Autodesk Inventor part; units mm, degrees
ref_plane "YZ Plane" through (0, 0, 0) normal (1, 0, 0) x (0, 1, 0)
ref_plane "XZ Plane" through (0, 0, 0) normal (0, 1, 0) x (-1, 0, 0)
ref_plane "XY Plane" through (0, 0, 0) normal (0, 0, 1) x (1, 0, 0)
sketch "Sketch1" plane through (0, 0, 0) normal (0, 0, 1) x (1, 0, 0)
  line L0 (0, 0) -> (0, 33)
  line L1 (0, 33) -> (19, 33)
  line L2 (19, 33) -> (19, 0)
  line L3 (19, 0) -> (0, 0)
  dimension "d0" = 33
  dimension "d1" = 19
extrude "Extrusion1" add sketch "Sketch1" along normal blind 4
sketch "Sketch2" plane through (0, 33, 0) normal (0, 1, 0) x (1, 0, 0)
  line L0 (19, 0) -> (0, 0)
  line L1 (19, 0) -> (19, -24)
  line L2 (19, -24) -> (15, -24)
  line L3 (15, -24) -> (15, 0)
  line L4 (15, 0) -> (19, 0)
  dimension "d4" = 24
  dimension "d5" = 4
  dimension "d6" = 24
extrude "Extrusion2" add sketch "Sketch2" against normal blind 33
sketch "Sketch3" plane through (0, 33, 0) normal (0, 1, 0) x (1, 0, 0)
  line L0 (15, -4) -> (15, -24)
  line L1 (15, -24) -> (95, -24)
  line L2 (95, -24) -> (95, -20)
  line L3 (95, -20) -> (15, -20)
  line L4 (15, -20) -> (15, -24)
  point P0 (0, 0)
  dimension "d9" = 80
  dimension "d10" = 4
  dimension "d11" = 80
extrude "Extrusion3" add sketch "Sketch3" against normal blind 33
sketch "Sketch4" plane through (0, 33, 0) normal (0, 1, 0) x (1, 0, 0)
  line L0 (15, -24) -> (95, -24)
  line L1 (95, -24) -> (95, 0)
  line L2 (95, 0) -> (91, 0)
  line L3 (91, 0) -> (91, -24)
  line L4 (91, -24) -> (95, -24)
  point P0 (0, 0)
  dimension "d14" = 24
  dimension "d15" = 4
  dimension "d16" = 24
extrude "Extrusion4" add sketch "Sketch4" against normal blind 33
sketch "Sketch5" plane through (0, 33, 0) normal (0, 1, 0) x (1, 0, 0)
  line L0 (91, 0) -> (91, -20)
  line L1 (91, 0) -> (110, 0)
  line L2 (110, 0) -> (110, -4)
  line L3 (110, -4) -> (91, -4)
  line L4 (91, -4) -> (91, 0)
  point P0 (0, 0)
  dimension "d19" = 19
  dimension "d20" = 4
  dimension "d21" = 19
  dimension "d22" = 4
extrude "Extrusion5" add sketch "Sketch5" against normal blind 33
sketch "Sketch6" plane through (15, 0, 24) normal (0, 0, 1) x (1, 0, 0)
  line L0 (80, 33) -> (80, 0)
  line L1 (30, 33) -> (30, 22.18)
  line L2 (50, 33) -> (50, 22.18)
  arc A0 (30.0006, 22.18) -> (49.9994, 22.18) centre (40, 16.5) ccw
  line L3 (30, 22.18) -> (30.0006, 22.18)
  line L4 (49.9994, 22.18) -> (50, 22.18)
  line L5 (30, 33) -> (50, 33)
  line L6 (0, 33) -> (80, 33)
  point P0 (-15, 0)
  dimension "d27" = 10.82
  dimension "d28" = 10.82
  dimension "d30" = 23
extrude "Extrusion6" cut sketch "Sketch6" against normal blind 4
sketch "Sketch7" plane through (0, 0, 0) normal (0, 0, -1) x (-1, 0, 0)
  line L0 (0, 33) -> (-19, 33)
  line L1 (-19, 0) -> (0, 0)
  circle A0 centre (-9.5, 24.5) radius 2.5
  circle A1 centre (-9.5, 8.5) radius 2.5
  dimension "d35" = 5
  dimension "d36" = 5
extrude "Extrusion7" cut sketch "Sketch7" against normal blind 4
sketch "Sketch8" plane through (91, 0, 0) normal (0, 0, -1) x (-1, 0, 0)
  circle A0 centre (-9.5, 24.5) radius 2.5
  circle A1 centre (-9.5, 8.5) radius 2.5
  point P0 (91, 0)
  point P1 (-19, 33)
  point P2 (0, 33)
  point P3 (-19, 0)
  point P4 (0, 0)
  dimension "d39" = 19
  dimension "d43" = 5
  dimension "d44" = 5
extrude "Extrusion8" cut sketch "Sketch8" against normal blind 4
sketch "Sketch9" plane through (15, 0, 24) normal (0, 0, 1) x (1, 0, 0)
  line L0 (0, 33) -> (30, 33)
  line L1 (0, 0) -> (0, 33)
  circle A0 centre (22.5, 16.5) radius 2.5
  line L2 (50, 33) -> (80, 33)
  line L3 (80, 0) -> (80, 33)
  circle A1 centre (57.5, 16.5) radius 2.5
  point P0 (-15, 0)
  dimension "d49" = 5
  dimension "d52" = 5
extrude "Extrusion9" cut sketch "Sketch9" against normal blind 4
sketch "Sketch10" plane through (0, 33, 0) normal (0, 1, 0) x (1, 0, 0)
  line L0 (31.4, -24) -> (31.4, -29.2)
  line L1 (31.4, -29.2) -> (35, -29.2)
  line L2 (37.6, -26.6) -> (37.6, -26.6)
  line L3 (40, -24) -> (35, -24)
  line L4 (35, -24) -> (31.4, -24)
  arc A0 (37.6, -26.6) -> (35, -24) centre (35, -26.6) ccw
  arc A1 (35, -29.2) -> (37.6, -26.6) centre (35, -26.6) ccw
  circle A2 centre (35, -26.6) radius 1.6
  point P0 (0, 0)
  point P1 (15, -24)
  point P2 (37.6, -29.2)
  point P3 (37.6, -24)
  dimension "d56" = 5.2
  dimension "d57" = 6.2
  dimension "d58" = 5.2
  dimension "d59" = 6.2
  dimension "d60" = 2.6
  dimension "d61" = 3.2
extrude "Extrusion10" add sketch "Sketch10" against normal blind 8
sketch "Sketch11" plane through (91, 33, 20) normal (0, 1, 0) x (1, 0, 0)
  line L0 (-12.4, -4) -> (-12.4, -9.2)
  line L1 (-12.4, -9.2) -> (-16, -9.2)
  line L2 (-18.6, -6.6) -> (-18.6, -6.6)
  line L3 (-16, -4) -> (-21, -4)
  line L4 (-16, -4) -> (-12.4, -4)
  arc A0 (-16, -4) -> (-18.6, -6.6) centre (-16, -6.6) ccw
  arc A1 (-18.6, -6.6) -> (-16, -9.2) centre (-16, -6.6) ccw
  circle A2 centre (-16, -6.6) radius 1.6
  point P0 (-91, 20)
  point P1 (4, -4)
  point P2 (-18.6, -9.2)
  point P3 (-18.6, -4)
  dimension "d64" = 16.4
  dimension "d65" = 5.2
  dimension "d66" = 6.2
  dimension "d67" = 5.2
  dimension "d68" = 6.2
  dimension "d69" = 2.6
  dimension "d70" = 3.2
extrude "Extrusion11" add sketch "Sketch11" against normal blind 8
For this review, take the finished solid that the model builds, in its own axes (mm). A direction names the side the tool comes from. Give positions to 0.01 mm unless a question says otherwise; leave off trailing zeros. Write each loop counter-clockwise with the first axis right and the second up, starting at its lowest first coordinate (ties: lowest second). Pieces come first, ordered by that corner, then holes.
Item 1: Wall thickness on probe 1 along X at (y, z) = (30.25, 26.6); probe 2 along X at (y, z) = (18, 12.75); probe 3 along X at (y, z) = (27.5, 21.25): over which ranges is each line inside the solid? List them lowest first.
Item 2: Insertion check: P1, Ø4.5, axis at x = 5.5, y = 21.5, coming from the +Z side; P2, Ø6, axis at y = 9, z = 17, coming from the -X side; P3, Ø10, axis at x = 12, z = 9, coming from the +Y side; P4, Ø1, axis at x = 34.5, y = 11.5, coming from the -Z side. Each pin has a flat end and moves straight along its axis. Give the tip position at first contact, or say it passes through.
Item 3: Machinability: for faces 5 (the face through (45, 28, 22)), 6 (the face through (48, 6, 20)), 7 (the face through (103, 17, 4)), 8 (the face through (77, 25, 27)), which of the approach directions +Z, -Z, +X, -X, +Y, -Y give a long, thin tool a straight path to every point of the face, cutting with its end or side? Answer none if there is none.
Item 4: Take a section at B-B (y = 16.5). Give the boundary of the cut face in (x, z), and give its area (3 significant figures).
Item 5: Take a section at D-D (z = 26.6). Give the boundary of the cut face in (x, y), and give its area (3 significant figures).
Item 6: Take a section at A-A (z = 2.5). Give the boundary of the cut face in (x, y), and give its area (3 significant figures).
Item 7: Take a section at C-C (z = 18.25). Give the boundary of the cut face in (x, y), and give its area (3 significant figures).
Item 8: The part is to be moulded in two halves that separate along X. For faces 1 (the face through (17, 33, 15)), 2 (the face through (99.16, 26.61, 1.97)), 3 (the face through (39.81, 15.54, 22.03)), 4 (the face through (15, 17, 14)), say which applies: +X half, -X half, draft (parallel to the pull), parting line (faces both ways), or undercut.
Established:
1. probe 1: x = 31.4 to 33.4, 36.6 to 37.6, 72.4 to 73.4, 76.6 to 78.6
1. probe 2: x = 15 to 19, 91 to 95
1. probe 3: x = 15 to 45, 65 to 95
2. P1: stops at z = 4
2. P2: stops at x = 15
2. P3: stops at y = 33
2. P4: stops at z = 20
3. face 5: +Z, -Z, +Y
3. face 6: -Z, +Y, -Y
3. face 7: +Z, +X, +Y, -Y
3. face 8: +Z, +X, -X, -Y
4. outline: (0, 0) - (19, 0) - (19, 20) - (35, 20) - (35, 24) - (15, 24) - (15, 4) - (0, 4) - close; (40, 20) - (43.5, 20) - (43.5, 24) - (40, 24) - close; (66.5, 20) - (70, 20) - (70, 24) - (66.5, 24) - close; (75, 20) - (91, 20) - (91, 0) - (110, 0) - (110, 4) - (95, 4) - (95, 24) - (75, 24) - close
4. area: 468 mm2
5. outline: (31.4, 25) - (33.4, 25) - (33.4, 33) - (31.4, 33) - close; (36.6, 25) - (37.6, 25) - (37.6, 33) - (36.6, 33) - close; (72.4, 25) - (73.4, 25) - (73.4, 33) - (72.4, 33) - close; (76.6, 25) - (78.6, 25) - (78.6, 33) - (76.6, 33) - close
5. area: 48.0 mm2
6. outline: (0, 0) - (19, 0) - (19, 33) - (0, 33) - close; (91, 0) - (110, 0) - (110, 33) - (91, 33) - close; hole circle Ø5 at (9.5, 8.5); hole circle Ø5 at (9.5, 24.5); hole circle Ø5 at (100.5, 8.5); hole circle Ø5 at (100.5, 24.5)
6. area: 1,180 mm2
7. outline: (15, 0) - (19, 0) - (19, 33) - (15, 33) - close; (91, 0) - (95, 0) - (95, 33) - (91, 33) - close
7. area: 264 mm2
8. face 1: draft
8. face 2: undercut
8. face 3: undercut
8. face 4: -X half
